Model file for the job. Use its own axes, mm. Face numbers are marked on the shaded views. Give positions to 0.01 mm unless a question says otherwise; leave off trailing zeros. Write each loop counter-clockwise with the first axis right and the second up, starting at its lowest first coordinate (ties: lowest second). Pieces come first, ordered by that corner, then holes. Notation, with made-up numbers: (-23, 83.5) - (-6, 83.5) arc R36 cw to (-6, 120.5) - close; hole circle Ø11 at (72, -11.75). An arc over 180 degrees is marked (long way). One line per item, written item: value. Start each with the question number.
(1) Cut at A-A, the plane x = -15. List the corners of the cut face in (y, z), and give its area (3 significant figures).
(2) Probe L1, parallel to Z at x = 15, y = 1.7; L2, parallel to X at y = 1.9, z = 91. List the from-to ranges inside material, lowest first.
(3) Mould opens along Z. For the marked faces 1, 2, 3 and 4 say: pulls with the +Z half, pulls with the -Z half, needs draft (parallel to the pull), parting line crosses it, or undercut.
(4) Cut at B-B, the plane z = 91. List the corners of the cut face in (x, y).
(5) Cut at C-C, the plane y = 1.5. List the corners of the cut face in (x, z).
from build123d import *

# Parameters (mm, degrees)
SKETCH048_W     = 40
SKETCH048_H     = 22
SKETCH048_R     = 1.65
PAD017_DEPTH    = 3
FILLET018_R     = 3
CHAMFER030_SIZE = 1


with BuildPart() as part:
    # Sketch048 → Pad017 (new body)
    with BuildSketch(Plane.XZ):
        with Locations((0, -11)):
            Rectangle(SKETCH048_W, SKETCH048_H)
        with Locations((15, -11)):
            Circle(SKETCH048_R, mode=Mode.SUBTRACT)
        with Locations((-15, -11)):
            Circle(SKETCH048_R, mode=Mode.SUBTRACT)
    extrude(amount=-PAD017_DEPTH)

    # Fillet018
    fillet018_edges = [part.edges().sort_by_distance(p)[0] for p in [
        (20, 1.5, 0),
        (-20, 1.5, 0),
    ]]
    fillet(fillet018_edges, radius=FILLET018_R)

    # Chamfer030
    chamfer030_edges = [part.edges().sort_by_distance(p)[0] for p in [
        (20, 1.5, -22),
        (-20, 1.5, -22),
    ]]
    chamfer(chamfer030_edges, length=CHAMFER030_SIZE)


with BuildPart() as part_1:
    # Body016 placement: moved
    add(part.part.moved(Location((0, 0.3, 102))))


solid = part_1.part
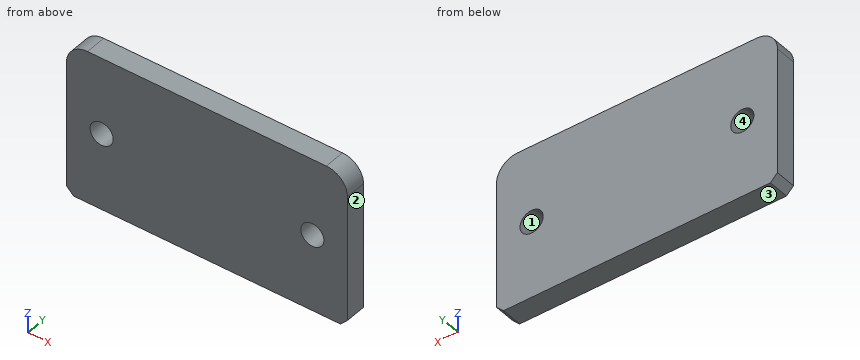
Answers follow:
1. outline: (0.3, 80) - (3.3, 80) - (3.3, 89.35) - (0.3, 89.35) - close; (0.3, 92.65) - (3.3, 92.65) - (3.3, 102) - (0.3, 102) - close
1. area: 56.1 mm²
2. L1: z = 80 to 89.35, 92.65 to 102
2. L2: x = -20 to -16.65, -13.35 to 13.35, 16.65 to 20
3. face 1: undercut
3. face 2: needs draft
3. face 3: pulls with the -Z half
3. face 4: undercut
4. outline: (-20, 0.3) - (-16.65, 0.3) - (-16.65, 3.3) - (-20, 3.3) - close; (-13.35, 0.3) - (13.35, 0.3) - (13.35, 3.3) - (-13.35, 3.3) - close; (16.65, 0.3) - (20, 0.3) - (20, 3.3) - (16.65, 3.3) - close
5. outline: (-20, 81) - (-19, 80) - (19, 80) - (20, 81) - (20, 99) arc R3 ccw to (17, 102) - (-17, 102) arc R3 ccw to (-20, 99) - close; hole circle Ø3.3 at (-15, 91); hole circle Ø3.3 at (15, 91)
